The drawing under review shows one solid part. Ordinate dimensions are in mm from its lowest x, y, z. A direction names the side the tool comes from. Give positions to 0.01 mm unless a question says otherwise; leave off trailing zeros. Order: outer loops, then holes, each group sorted by start corner. A loop starts at its lowest first (then second) coordinate and runs counter-clockwise, first axis right, second up. Notation, with made-up numbers: (2, 32) -> (37, 32) arc R20 ccw to (37, 45) -> close; hole circle Ø3 at (55, 20). An arc over 180 degrees is marked (long way). One line per item, written item: value.
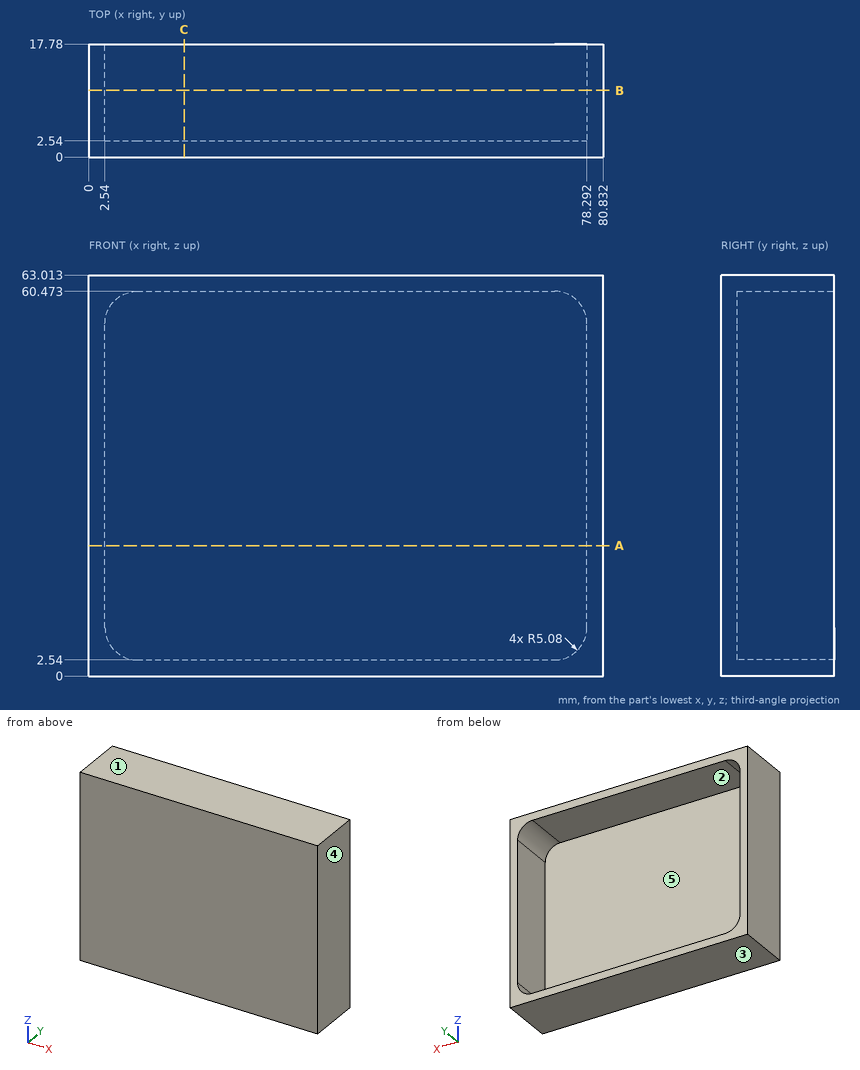
Item 1: Draft analysis for pull direction Z (two halves, no side actions). For the marked faces 1, 2 and 3, state which applies: pulls with the +Z half, pulls with the -Z half, needs draft (parallel to the pull), parting line crosses it, or undercut.
Returned:
face 1: pulls with the +Z half
face 2: undercut
face 3: pulls with the -Z half
Item 2: Clearance check with flat-ended pins moving along their axes: P1, Ø4, axis at x = 45.5, z = 47, coming from the +Y side; P2, Ø4.5, axis at x = 51.5, y = 7, coming from the -Z side. State where each tip first meets the part, or that it passes through.
Returned:
P1: y = 2.54
P2: z = 0
Item 3: Machinability: for the marked faces 4 and 5, which of the approach directions +Z, -Z, +X, -X, +Y, -Y give a long, thin tool a straight path to every point of the face, cutting with its end or side? Answer none if there is none.
Returned:
face 4: +Z, -Z, +X, +Y, -Y
face 5: +Y
Item 4: To check wall thickness, follow line 1 along X through (y, z) = (8.25, 16); line 2 along Z through (x, y) = (40.5, 14.5); line 3 along Y through (x, z) = (35, 41.5). State the ranges of each line that lie inside material, in increasing order. Write a range as from..to.
Returned:
line 1: 0..2.54, 78.29..80.83
line 2: 0..2.54, 60.47..63.01
line 3: 0..2.54
Item 5: Add section C-C on x = 15. Give the boundary of the cut face in (y, z).
Returned:
outline: (0, 0) -> (17.78, 0) -> (17.78, 2.54) -> (2.54, 2.54) -> (2.54, 60.47) -> (17.78, 60.47) -> (17.78, 63.01) -> (0, 63.01) -> close
Item 6: Add section B-B on y = 10.5. Give the boundary of the cut face in (x, z).
Returned:
outline: (0, 0) -> (80.83, 0) -> (80.83, 63.01) -> (0, 63.01) -> close; hole (2.54, 7.62) arc R5.08 ccw to (7.62, 2.54) -> (73.21, 2.54) arc R5.08 ccw to (78.29, 7.62) -> (78.29, 55.39) arc R5.08 ccw to (73.21, 60.47) -> (7.62, 60.47) arc R5.08 ccw to (2.54, 55.39) -> close
Item 7: Add section A-A on z = 20.5. Give the boundary of the cut face in (x, y).
Returned:
outline: (0, 0) -> (80.83, 0) -> (80.83, 17.78) -> (78.29, 17.78) -> (78.29, 2.54) -> (2.54, 2.54) -> (2.54, 17.78) -> (0, 17.78) -> close
